Part model, mm, in its own coordinate system. Face numbers are marked on the shaded views. A direction names the side the tool comes from. Coordinates: 2 decimals unless noted, no trailing zeros. Loops run counter-clockwise (first coordinate to the right, second up) from the corner with the lowest first, then second, coordinate; pieces in that order, holes last. Notation, with made-up numbers: (54.5, 72.25) - (109.5, 72.25) arc R30 cw to (109.5, 110.25) - close; hole circle Ø2 at (62.5, -27). An arc over 180 degrees is marked (long way). Use a Markdown table: item, result. Add a question column.
1) Band-saw the part on D-D (z = 2.5). Give the cut face in (x, y), plus the area to 3 significant figures.
2) Pull direction X, two halves, no side cores. Call the marked faces 3 and 4: +X half, -X half, draft (parallel to the pull), parting line (faces both ways), or undercut.
3) Drop flat-ended pins along their axis: P1, Ø12, axis at y = -12, z = 18.5, coming from the +X side; P2, Ø12, axis at x = 10, z = 10.5, coming from the +Y side; P3, Ø4, axis at y = 9, z = 7, coming from the -X side. Give the stop position or say it passes through.
4) Band-saw the part on C-C (z = 7.5). Give the cut face in (x, y) (1 decimal), plus the area to 3 significant figures.
5) Tool access for the marked faces 1 and 2: list every direction of +Z, -Z, +X, -X, +Y, -Y with a clear straight run to the whole face (end or side of a thin tool).
6) Probe probe 1 along Z at (x, y) = (8, -1.5) (3 decimals); probe 2 along Y at (x, z) = (0, 10); probe 3 along X at (y, z) = (4, 8). List the from-to ranges inside material, lowest first. Write a range as [from, to].
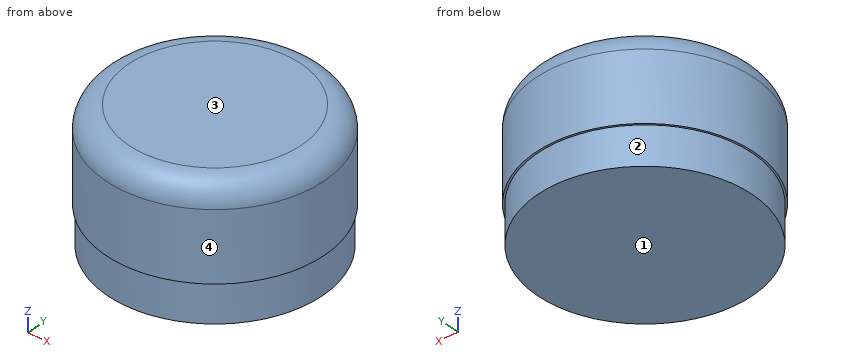
from build123d import *

# Parameters (mm, degrees)
F1_R     = 18.0975
F2_DEPTH = 15.24
F3_R     = 3.81
F5_T     = -1.905
F4_R     = 17.78
F6_DEPTH = 6.35


with BuildPart() as f2:
    # F1 (on offset) → F2 (new body)
    with BuildSketch(Plane.XY.offset(6.35)):
        Circle(F1_R)
    extrude(amount=F2_DEPTH)

    # F3
    f3_edges = [f2.edges().sort_by_distance(p)[0] for p in [
        (-18.0975, 0, 21.59),
    ]]
    fillet(f3_edges, radius=F3_R)

    # F5
    f5_openings = [f2.faces().sort_by_distance(p)[0] for p in [
        (0, 0, 6.35),
    ]]
    offset(amount=F5_T, openings=f5_openings)

    # F4 (on Top) → F6 (join)
    with BuildSketch(Plane.XY):
        Circle(F4_R)
    extrude(amount=F6_DEPTH)


solid = f2.part
Answer block:
| question | item | result |
|---|---|---|
| 1 | outline | circle Ø35.56 at (0, 0) |
| 1 | area | 993 mm2 |
| 2 | face 3 | draft |
| 2 | face 4 | parting line |
| 3 | P1 | x = 17.06 |
| 3 | P2 | y = 17.65 |
| 3 | P3 | x = -16.69 |
| 4 | outline | circle Ø36.2 at (0, 0); hole circle Ø32.4 at (0, 0) |
| 4 | area | 205 mm2 |
| 5 | face 1 | -Z, +X, -X, +Y, -Y |
| 5 | face 2 | -Z |
| 6 | probe 1 | [0, 6.35], [19.685, 21.59] |
| 6 | probe 2 | [-18.1, -16.19], [16.19, 18.1] |
| 6 | probe 3 | [-17.65, -15.69], [15.69, 17.65] |
